from build123d import *

# Parameters (mm, degrees)
F1_DEPTH = 63.5
F0_W     = 25.4
F0_H     = 19.05
F2_DEPTH = 25.4
F3_DEPTH = 7.9375
F5_R     = 6.35


# Not quite as in the source:
# - a feature of the source that left no trace in its solid (it failed there, or was rolled back) is left out


with BuildPart() as f1:
    # F0 (on Front) → F1 (new body, symmetric)
    with BuildSketch(Plane.XZ):
        Polygon((22.225, 9.525), (-41.275, 9.525), (-41.275, -9.525), (41.275, -9.525), (41.275, 9.525), align=None)
    extrude(amount=F1_DEPTH, both=True)

    # F0 (on Front) → F2 (join, symmetric)
    with BuildSketch(Plane.XZ):
        with BuildLine():
            Line((22.225, 27.0002), (22.225, 9.525))
            Line((22.225, 9.525), (41.275, 9.525))
            Line((41.275, 9.525), (41.275, 27.0002))
            ThreePointArc((41.275, 27.0002), (45.9246798487, 38.2255201513), (57.15, 42.8752))
            Line((57.15, 42.8752), (60.325, 42.8752))
            Line((60.325, 42.8752), (60.325, 61.9252))
            Line((60.325, 61.9252), (57.15, 61.9252))
            add(Edge.make_bspline(
                [(53.8854342407, 61.7722898912), (54.9842067368, 61.8365871986), (56.0728453275, 61.8876096574), (57.15, 61.9252)],
                knots=[108.5245810491, 108.5245810491, 108.5245810491, 108.5245810491, 111.5045361635, 111.5045361635, 111.5045361635, 111.5045361635], degree=3))
            ThreePointArc((53.8854342407, 61.7722898912), (31.3258777096, 50.5133948686), (22.225, 27.0002))
        make_face()
        with Locations((73.025, 52.4002)):
            Rectangle(F0_W, F0_H)
    extrude(amount=F2_DEPTH, both=True)

    # F0 (on Front) → F3 (join, symmetric)
    with BuildSketch(Plane.XZ):
        with BuildLine():
            add(Edge.make_bspline(
                [(-41.275, 9.525), (-39.5856284224, 39.4828766469), (13.870125209, 59.4306981306), (53.8854342407, 61.7722898912)],
                knots=[0, 0, 0, 0, 108.5245810491, 108.5245810491, 108.5245810491, 108.5245810491], degree=3))
            Line((-41.275, 9.525), (22.225, 9.525))
            Line((22.225, 9.525), (22.225, 27.0002))
            ThreePointArc((22.225, 27.0002), (31.3258777096, 50.5133948686), (53.8854342407, 61.7722898912))
        make_face()
    extrude(amount=F3_DEPTH, both=True)

    # F0 (on Front) → F4 (revolve)
    with BuildSketch(Plane.XZ):
        Polygon((85.725, 66.675), (85.725, 61.9252), (85.725, 42.8752), (85.725, 38.1), (111.125, 38.1), (111.125, 66.675), align=None)
    revolve(axis=Axis((85.725, 0, 52.3875), (0, 0, 1)))

    # F5
    f5_edges = [f1.edges().sort_by_distance(p)[0] for p in [
        (-41.275, -63.5, 0),
        (41.275, -63.5, 0),
        (-41.275, 63.5, 0),
        (41.275, 63.5, 0),
    ]]
    fillet(f5_edges, radius=F5_R)


solid = f1.part
Check sheet for the modelled part. Datum: model origin and axes. Units: mm. A direction names the side the tool comes from. Round coordinates to 2 decimals unless told otherwise and drop trailing zeros. Write each loop counter-clockwise with the first axis right and the second up, starting at its lowest first coordinate (ties: lowest second). Pieces come first, ordered by that corner, then holes. Notation, with made-up numbers: (57.25, 2) -> (108.25, 2) arc R27 cw to (108.25, 22) -> close; hole circle Ø6 at (19.5, 69.5). An arc over 180 degrees is marked (long way). Answer as CSV lines item,"result". Start each with the question number.
1) Go/stop test with flat-tipped pins: P1, Ø18.5, axis at y = -11.5, z = 2.5, coming from the +X side (3 decimals); P2, Ø8.5, axis at y = 17, z = 22.5, coming from the -X side (3 decimals); P3, Ø8, axis at x = 48.5, z = 43, coming from the -Y side. Record where each tip stops, or that it passes through.
2) Release check for a two-part mould opening along X. For faces 5 (the cylindrical face through (39.464, -61.59, 0.133)), 6 (the flat face through (60, 2, 42.875)), 7 (the cylindrical face through (31.57, -16.79, 50.78)), 8 (the flat face through (0, -63.5, 0)) record: pulls with the +X half, pulls with the -X half, needs draft (parallel to the pull), parting line crosses it, or undercut.
3) Section check A-A on z = -2. Enter the section's corners in (x, y) (3 decimals), and give its area (3 significant figures).
4) Section check B-B on x = 68. Enter the section's corners in (y, z) (3 decimals), and give its area (3 significant figures).
5) Section check C-C on x = 91.5. Enter the section's corners in (y, z) (3 decimals), and give its area (3 significant figures).
6) Material ranges on line 1 (Z direction, x = 82, y = 1) (3 decimals); line 2 (Z direction, x = -23, y = -11) (3 decimals); line 3 (X direction, y = -39, z = -1.5) (3 decimals), recorded low to high. Write a range as from..to.
7) Tool access check on faces 1 (the flat face through (46, 25.4, 42)), 2 (the cylindrical face through (-39.464, 61.59, -0.133)), 3 (the flat face through (-4, 7.938, 30)), 4 (the flat face through (-4, -7.938, 30)). Record the directions out of +Z, -Z, +X, -X, +Y, -Y that give a thin tool (end or side, any length) a straight path to the whole face; none if there is none.
Found:
1,P1,"stops at x = 41.275"
1,P2,"stops at x = 22.225"
1,P3,"stops at y = -25.4"
2,face 5,"pulls with the +X half"
2,face 6,"undercut"
2,face 7,"pulls with the -X half"
2,face 8,"needs draft"
3,outline,"(-41.275, -57.15) arc R6.35 ccw to (-34.925, -63.5) -> (34.925, -63.5) arc R6.35 ccw to (41.275, -57.15) -> (41.275, 57.15) arc R6.35 ccw to (34.925, 63.5) -> (-34.925, 63.5) arc R6.35 ccw to (-41.275, 57.15) -> close"
3,area,"10,400 mm^2"
4,outline,"(-25.4, 42.875) -> (-18.193, 42.875) -> (-18.193, 38.1) -> (18.193, 38.1) -> (18.193, 42.875) -> (25.4, 42.875) -> (25.4, 61.925) -> (18.193, 61.925) -> (18.193, 66.675) -> (-18.193, 66.675) -> (-18.193, 61.925) -> (-25.4, 61.925) -> close"
4,area,"1,310 mm^2"
5,outline,"(-24.735, 38.1) -> (24.735, 38.1) -> (24.735, 66.675) -> (-24.735, 66.675) -> close"
5,area,"1,410 mm^2"
6,line 1,"z = 38.1..66.675"
6,line 2,"z = -9.525..9.525"
6,line 3,"x = -41.275..41.275"
7,face 1,"+Z, +X, -X, +Y"
7,face 2,"+Z, -Z, -X, +Y"
7,face 3,"+Z, -X, +Y"
7,face 4,"+Z, -X, -Y"
